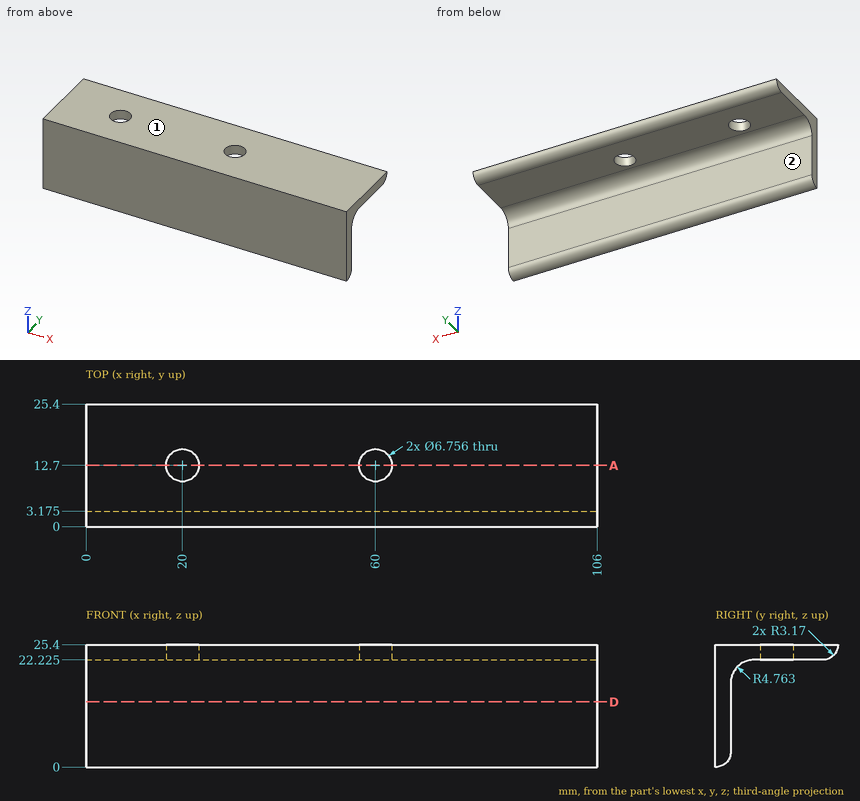
The figure shows three views and two pictorial views of one solid part (mm, origin at its lowest corner). Answer the questions. A direction names the side the tool comes from. Coordinates: 2 decimals unless noted, no trailing zeros. Write each loop counter-clockwise with the first axis right and the second up, starting at its lowest first coordinate (ties: lowest second). Pieces come first, ordered by that corner, then holes. Notation, with made-up numbers: M 49.5,26.5 L 77.5,26.5 A29 ccw 77.5,54.5 Z; hole C 22.25,23.5 d3. An arc over 180 degrees is marked long. Answer as CSV lines item,"result". Start each with the question number.
Item 1: A tool of negligible diameter and unlimited length cuts with its end or side. For the marked faces 1 and 2, from which of +Z, -Z, +X, -X, +Y, -Y can it reach the whole face along a straight path? Write none if from no direction.
Item 2: Consider L1, parallel to Y at x = 9.5, z = 11.5 (1 decimal); L2, parallel to Z at x = 72, y = 22 (1 decimal); L3, parallel to Y at x = 60, z = 23.7. Determine where each line is inside the solid, lowest interval first.
Item 3: Section D-D on z = 13.5 is taken. Write down the section's boundary in (x, y) (1 decimal).
Item 4: Flat-ended cylindrical pins translate along their axes: P1, Ø4, axis at x = 46.5, z = 8, coming from the -Y side; P2, Ø1, axis at x = 50, z = 5.5, coming from the +Y side (1 decimal); P3, Ø12, axis at x = 94.5, y = 19, coming from the -Z side (1 decimal). Find the tip coordinate at first contact, or state that the pin passes through.
Item 5: Section A-A on y = 12.7 is taken. Write down the section's boundary in (x, z) (1 decimal).
Checks:
1,face 1,"+Z, +X, -X, +Y, -Y"
1,face 2,"-Z, +X, -X, +Y"
2,L1,"y = 0 to 3.2"
2,L2,"z = 22.2 to 25.4"
2,L3,"y = 0 to 9.32, 16.08 to 24.91"
3,outline,"M 0,0 L 106,0 L 106,3.2 L 0,3.2 Z"
4,P1,"stops at y = 0"
4,P2,"stops at y = 3.2"
4,P3,"stops at z = 22.2"
5,outline,"M 0,22.2 L 16.6,22.2 L 16.6,25.4 L 0,25.4 Z; M 23.4,22.2 L 56.6,22.2 L 56.6,25.4 L 23.4,25.4 Z; M 63.4,22.2 L 106,22.2 L 106,25.4 L 63.4,25.4 Z"
